Read the model definition and answer for the solid it produces. Units are mm, in the model's axes. A direction names the side the tool comes from. Coordinates: 2 decimals unless noted, no trailing zeros. Loops run counter-clockwise (first coordinate to the right, second up) from the corner with the lowest first, then second, coordinate; pieces in that order, holes last. Notation, with made-up numbers: M 22,4 L 62,4 A28 cw 62,30 Z; hole C 45.5,7.25 d5. An arc over 180 degrees is marked long. Put each result on its own line as item: value.
from build123d import *

# Parameters (mm, degrees)
SKETCH1_R         = 7.112
SKETCH1_R_2       = 4.00812
EXTRUDE1_DEPTH    = 6.604
EXTRUDE2_DEPTH    = 6.604
CIRPATTERN1_COUNT = 12
EXTRUDE3_DEPTH    = 14.208


with BuildPart() as part:
    # Sketch1 → Extrude1 (new body, symmetric)
    with BuildSketch(Plane.XY):
        Circle(SKETCH1_R)
        Circle(SKETCH1_R_2, mode=Mode.SUBTRACT)
    extrude(amount=EXTRUDE1_DEPTH, both=True)

    # Sketch2 → Extrude2 (add, symmetric)
    with BuildSketch(Plane.XY):
        with BuildLine():
            ThreePointArc((-1.223214196, 7.006018201), (0, 7.112), (1.223214196, 7.006018201))
            ThreePointArc((1.223214196, 7.006018201), (1.000294904, 8.346410328), (0.569675744, 9.635173768))
            ThreePointArc((0.569675744, 9.635173768), (0, 9.652), (-0.569675744, 9.635173768))
            ThreePointArc((-0.569675744, 9.635173768), (-1.000294904, 8.346410328), (-1.223214196, 7.006018201))
        make_face()
    extrude2 = extrude(amount=EXTRUDE2_DEPTH, both=True)

    # CirPattern1: Extrude2 ×12 about axis
    cirpattern1_axis = Axis((0, 0, 0), (0, 0, 1))
    for i in range(1, CIRPATTERN1_COUNT):
        add(extrude2.rotate(cirpattern1_axis, i * 360 / CIRPATTERN1_COUNT))

    # Sketch3 → Extrude3 (cut, through all)
    with BuildSketch(Plane.XY.offset(6.604)):
        with BuildLine():
            Line((-1.0414, 3.870466635), (-1.0414, 5.04825))
            Line((-1.0414, 5.04825), (1.0414, 5.04825))
            Line((1.0414, 5.04825), (1.0414, 3.870466635))
            ThreePointArc((1.0414, 3.870466635), (0, 4.00812), (-1.0414, 3.870466635))
        make_face()
    extrude(amount=-EXTRUDE3_DEPTH, mode=Mode.SUBTRACT)


solid = part.part
1) Straight lines are drawn through the part: line 1 (Y direction, x = -7.75, z = -3); line 2 (X direction, y = -7.25, z = 4.75); line 3 (X direction, y = -8.25, z = -6). For each, find the intervals that lie inside material, in ascending order. Write a range as [from, to].
Answer list:
line 1: y = [-5.27, -3.33], [-1.13, 1.13], [3.33, 5.27]
line 2: x = [-5.17, -2.88], [-1.2, 1.2], [2.88, 5.17]
line 3: x = [-5.01, -3.86], [-1.02, 1.02], [3.86, 5.01]
2) Given pin 1 Ø0.9 at (y, z) = (4.5, 2) entering from +X; pin 2 Ø2 at (y, z) = (-3, 5) entering from -X; pin 3 Ø2 at (y, z) = (-7, 2.5) entering from +X, each flat-ended and moving along its own axis, determine where each tip first touches the part or whether it passes through.
Answer list:
pin 1: stops at x = 8.63
pin 2: stops at x = -8.37
pin 3: stops at x = 5.3
3) Find section A-A, the plane y = 0. Write down the section's boundary in (x, z), plus the area to 3 significant figures.
Answer list:
outline: M -9.65,-6.6 L -4.01,-6.6 L -4.01,6.6 L -9.65,6.6 Z; M 4.01,-6.6 L 9.65,-6.6 L 9.65,6.6 L 4.01,6.6 Z
area: 149 mm^2
4) Find section B-B, the plane x = 0. Write down the section's boundary in (y, z).
Answer list:
outline: M -9.65,-6.6 L -4.01,-6.6 L -4.01,6.6 L -9.65,6.6 Z; M 5.05,-6.6 L 9.65,-6.6 L 9.65,6.6 L 5.05,6.6 Z
5) Find section C-C, the plane x = -7.75. Write down the section's boundary in (y, z).
Answer list:
outline: M -5.27,-6.6 L -3.33,-6.6 L -3.33,6.6 L -5.27,6.6 Z; M -1.13,-6.6 L 1.13,-6.6 L 1.13,6.6 L -1.13,6.6 Z; M 3.33,-6.6 L 5.27,-6.6 L 5.27,6.6 L 3.33,6.6 Z
6) Determine the mould class of faces 5 (the cylindrical face through (3.29, -7.71, 0.09)), 6 (the cylindrical face through (-6.71, 5.034, 0.092)), 7 (the cylindrical face through (-5.045, 6.746, 0.092)) for opening direction Y: released by +Y, released by -Y, zero draft, split by the parting line, or undercut.
Answer list:
face 5: released by -Y
face 6: released by +Y
face 7: undercut
7) Which of the six approach directions +Z, -Z, +X, -X, +Y, -Y give full straight-line access (tool end or side, diameter ignored) to faces 1 (the cylindrical face through (-1.832, 6.872, 0.092)), 2 (the cylindrical face through (-5.04, -5.02, 0.09)), 3 (the cylindrical face through (-8.328, 1.005, 0.092)), 4 (the cylindrical face through (8.328, -1.005, 0.092))?
Answer list:
face 1: +Z, -Z, +Y
face 2: +Z, -Z
face 3: +Z, -Z, -X
face 4: +Z, -Z, +X
